```python
from build123d import *

# Parameters (mm, degrees)
ESQUISSE1_W             = 4
ESQUISSE1_H             = 85
BOSS_EXTRU_1_DEPTH      = 22.93
BOSS_EXTRU_5_DEPTH      = 22.9
ESQUISSE5_W             = 25.35
ESQUISSE5_H             = 21.181614094
BOSS_EXTRU_6_DEPTH      = 4
CONG_1_R                = 2
CONG_5_R                = 1
ESQUISSE9_R             = 1.8
ENL_V_MAT_EXTRU_1_DEPTH = 58
BOSS_EXTRU_8_DEPTH      = 1
BOSS_EXTRU_9_DEPTH      = 22.9


with BuildPart() as part:
    # Esquisse1 → Boss.-Extru.1 (new body)
    with BuildSketch(Plane.XY):
        with Locations((-2, -15.95097561)):
            Rectangle(ESQUISSE1_W, ESQUISSE1_H)
    extrude(amount=BOSS_EXTRU_1_DEPTH)

    # Esquisse2 → Boss.-Extru.5 (add)
    with BuildSketch(Plane.XY.offset(22.93)):
        Polygon((-33.850627534, 38.869645224), (0, 26.54902439), (0, 22.54902439), (-4, 22.54902439), (-35.604113867, 34.051981118), align=None)
    extrude(amount=-BOSS_EXTRU_5_DEPTH)

    # Esquisse5 → Boss.-Extru.6 (add)
    with BuildSketch(Plane.XY.offset(22.93)):
        with Locations((-12.675, -32.061782657)):
            Rectangle(ESQUISSE5_W, ESQUISSE5_H)
    extrude(amount=-BOSS_EXTRU_6_DEPTH)

    # Congé1
    cong_1_edges = [part.edges().sort_by_distance(p)[0] for p in [
        (-2, -58.45097561, 22.93),
        (-2, -58.45097561, 0),
    ]]
    fillet(cong_1_edges, radius=CONG_1_R)

    # Congé5
    cong_5_edges = [part.edges().sort_by_distance(p)[0] for p in [
        (-14.675, -21.47097561, 22.93),
        (-14.675, -42.652589704, 22.93),
    ]]
    fillet(cong_5_edges, radius=CONG_5_R)

    # Esquisse9 → Enlèv. mat.-Extru.1 (cut)
    with BuildSketch(Plane(origin=(0, 0, 0), x_dir=(1, 0, 0), z_dir=(0, 1, 0))):
        with Locations((-24.9342899, -11.439091382)):
            Circle(ESQUISSE9_R)
        with Locations((-8.483694977, -11.459545691)):
            Circle(ESQUISSE9_R)
    extrude(amount=ENL_V_MAT_EXTRU_1_DEPTH, mode=Mode.SUBTRACT)

    # Esquisse10 → Boss.-Extru.8 (add)
    with BuildSketch(Plane.ZY.offset(4)):
        with BuildLine():
            Line((10.166030362, 18.2390183), (11.166631323, 18.2390183))
            add(Edge.make_bspline(
                [(11.166631323, 18.2390183), (11.233404364, 18.238796034), (11.361615999, 18.238369259), (11.545292099, 18.235989598), (11.712187952, 18.22916909), (11.862216294, 18.223299685), (11.995374373, 18.212596912), (12.112070502, 18.202367416), (12.211767213, 18.188976472), (12.272118429, 18.176540153), (12.299443823, 18.170909326)],
                knots=[0, 0, 0, 0, 0.000200323, 0.000384642, 0.000551017, 0.000701421, 0.00083501, 0.000951717, 0.001052854, 0.001136534, 0.001136534, 0.001136534, 0.001136534], degree=3))
            add(Edge.make_bspline(
                [(12.299443823, 18.170909326), (12.336024715, 18.161871089), (12.408406128, 18.143987427), (12.512620508, 18.106187997), (12.611926685, 18.062445676), (12.705912149, 18.011068933), (12.794106136, 17.951676391), (12.877418009, 17.885293359), (12.956225814, 17.812283065), (13.027342428, 17.73080472), (13.094398216, 17.645323991), (13.150953397, 17.552890053), (13.199705511, 17.456230728), (13.238520535, 17.354362988), (13.269774783, 17.248274743), (13.291812268, 17.137005033), (13.30502825, 17.021060783), (13.306373758, 16.941978056), (13.307056003, 16.901878877)],
                knots=[0, 0, 0, 0, 0.000112973, 0.000223535, 0.000332046, 0.000438282, 0.0005444, 0.000650613, 0.000757615, 0.000866163, 0.000974744, 0.001083144, 0.001190647, 0.001299089, 0.001409706, 0.001522064, 0.001638977, 0.001759236, 0.001759236, 0.001759236, 0.001759236], degree=3))
            add(Edge.make_bspline(
                [(13.307056003, 16.901878877), (13.304957434, 16.835257299), (13.300862583, 16.705261345), (13.262683863, 16.516602943), (13.200145978, 16.340618207), (13.113969851, 16.177528725), (13.004227743, 16.030513517), (12.872335184, 15.901384295), (12.718218596, 15.793327277), (12.574748145, 15.718394699), (12.448013574, 15.67040483), (12.34368027, 15.636638603), (12.229870302, 15.610550081), (12.10767411, 15.587178464), (11.976583173, 15.569533186), (11.836911688, 15.55660948), (11.688560043, 15.548532268), (11.586647087, 15.547329403), (11.534219464, 15.546710608)],
                knots=[0, 0, 0, 0, 0.000199681, 0.000389629, 0.000574641, 0.000758347, 0.00094084, 0.00112287, 0.00130963, 0.001503603, 0.001606651, 0.001715936, 0.001832303, 0.001956651, 0.002089094, 0.002228924, 0.002377378, 0.002534658, 0.002534658, 0.002534658, 0.002534658], degree=3))
            Line((11.534219464, 15.546710608), (13.371158567, 13.2390183))
            Line((13.371158567, 13.2390183), (12.816270746, 13.2390183))
            Line((12.816270746, 13.2390183), (10.979331644, 15.546710608))
            Line((10.979331644, 15.546710608), (10.61474831, 15.546710608))
            Line((10.61474831, 15.546710608), (10.61474831, 13.2390183))
            Line((10.61474831, 13.2390183), (10.166030362, 13.2390183))
            Line((10.166030362, 13.2390183), (10.166030362, 18.2390183))
        make_face()
        with BuildLine():
            Line((10.61474831, 17.726197787), (10.61474831, 16.05953112))
            Line((10.61474831, 16.05953112), (11.530213054, 16.052519902))
            add(Edge.make_bspline(
                [(11.530213054, 16.052519902), (11.572955967, 16.052500993), (11.655803905, 16.052464341), (11.775661998, 16.058169736), (11.887262158, 16.06466019), (11.990177518, 16.074587827), (12.084454054, 16.087382215), (12.170044644, 16.103386478), (12.247089004, 16.122032282), (12.336944059, 16.150891747), (12.437281961, 16.196614631), (12.546326904, 16.263136772), (12.639187386, 16.346806942), (12.717641475, 16.442483308), (12.78068352, 16.547677949), (12.825129312, 16.661129905), (12.853332801, 16.779975045), (12.856659294, 16.861658056), (12.858338054, 16.902880479)],
                knots=[0, 0, 0, 0, 0.000128209, 0.000248506, 0.000359904, 0.000463555, 0.000558601, 0.000645233, 0.000724669, 0.000796254, 0.000928055, 0.001054503, 0.00117794, 0.001301056, 0.001424562, 0.001544156, 0.0016654, 0.001788926, 0.001788926, 0.001788926, 0.001788926], degree=3))
            add(Edge.make_bspline(
                [(12.858338054, 16.902880479), (12.856620738, 16.94308987), (12.853217645, 17.022770211), (12.82543369, 17.139421512), (12.778448859, 17.249517155), (12.715131376, 17.352609276), (12.637989726, 17.446188899), (12.547535708, 17.52625626), (12.446242572, 17.592326924), (12.351569432, 17.634547468), (12.266949128, 17.660432973), (12.193478185, 17.678648921), (12.110461789, 17.693283876), (12.017496848, 17.705009678), (11.914980232, 17.715088169), (11.802393588, 17.721876425), (11.680483902, 17.725896231), (11.595988286, 17.726094929), (11.55224831, 17.726197787)],
                knots=[0, 0, 0, 0, 0.00012053, 0.000238846, 0.000357345, 0.000478278, 0.000600621, 0.000719816, 0.000839275, 0.000962126, 0.001029286, 0.001104593, 0.001189072, 0.001282, 0.00138565, 0.001498049, 0.00162031, 0.001751524, 0.001751524, 0.001751524, 0.001751524], degree=3))
            Line((11.55224831, 17.726197787), (10.61474831, 17.726197787))
        make_face(mode=Mode.SUBTRACT)
    extrude(amount=BOSS_EXTRU_8_DEPTH)

    # Esquisse11 → Boss.-Extru.9 (add)
    with BuildSketch(Plane.XY.offset(22.93)):
        Polygon((-5.452843765, 23.077816276), (-4, 20.298440223), (-0.659211444, 23.077816276), align=None)
    extrude(amount=-BOSS_EXTRU_9_DEPTH)


solid = part.part
```
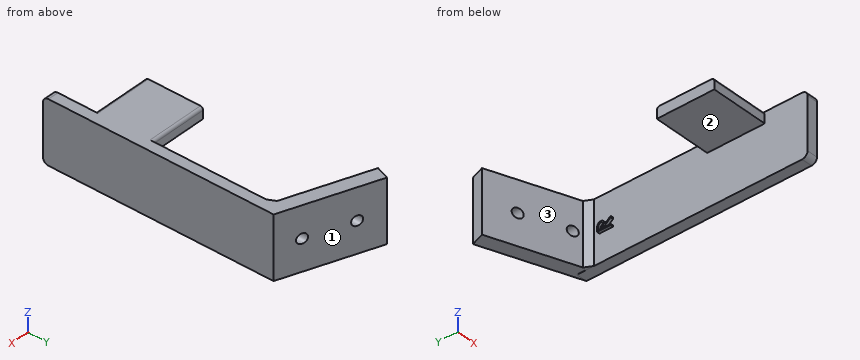
For this review, take the finished solid that the model builds, in its own axes (mm). Face numbers are marked on the shaded views. A direction names the side the tool comes from. Give positions to 0.01 mm unless a question says otherwise; leave off trailing zeros. Order: outer loops, then holes, each group sorted by start corner. A loop starts at its lowest first (then second) coordinate and runs counter-clockwise, first axis right, second up.
1) Wall thickness on line 1 (X direction, y = -27, z = 1.75); line 2 (X direction, y = -31, z = 19.5); line 3 (Z direction, x = -16.5, y = -27.5): over which ranges is each line inside the solid? List them lowest first.
2) Take a section at C-C (y = 27.5). Give the boundary of the cut face in (x, z), then the cut area to 3 significant figures.
3) Take a section at A-A (z = 4.5). Give the boundary of the cut face in (x, y).
4) Take a section at B-B (x = -13). Give the boundary of the cut face in (y, z).
5) For the marked faces 1, 2 and 3, list the 3-axis set-ups (+Z, -Z, +X, -X, +Y, -Y) from which the entire face can be reached by the end or side of a thin tool; tool diameter is ignored.
6) Insertion check: pin 1 (1.1 mm diameter, centred on x = -4.5, z = 10.5, fed in from +Y); pin 2 (5 mm diameter, centred on y = 2, z = 17, fed in from -X); pin 3 (2 mm diameter, centred on y = 11.5, z = 6.5, fed in from +X); pin 4 (1.8 mm diameter, centred on y = 17, z = 12, fed in from -X). Each pin has a flat end and moves straight along its axis. Give the tip position at first contact, or say it passes through.
Derived:
1. line 1: x = -4 to 0
1. line 2: x = -25.35 to 0
1. line 3: z = 18.93 to 22.93
2. outline: (-17.6, 0.03) - (-2.61, 0.03) - (-2.61, 22.93) - (-17.6, 22.93) - close; hole circle Ø3.6 at (-8.48, 11.46)
2. area: 333 mm2
3. outline: (-35.6, 34.05) - (-5.45, 23.08) - (-4, 20.3) - (-4, -58.45) - (0, -58.45) - (0, 26.55) - (-33.85, 38.87) - close
4. outline: (-42.65, 18.93) - (-21.47, 18.93) - (-21.47, 21.93) arc R1 ccw to (-22.47, 22.93) - (-41.65, 22.93) arc R1 ccw to (-42.65, 21.93) - close; (25.82, 0.03) - (31.28, 0.03) - (31.28, 22.93) - (25.82, 22.93) - close
5. face 1: +Z, -Z, +X, +Y
5. face 2: -Z, -X, -Y
5. face 3: +Z, -Z, -X
6. pin 1: stops at y = 28.39
6. pin 2: stops at x = -4
6. pin 3: stops at x = 0
6. pin 4: stops at x = -5
